Job drawing, mm, ordinate dimensions from the low corner. One solid piece. Coordinates: 2 decimals unless noted, no trailing zeros. Write each loop counter-clockwise with the first axis right and the second up, starting at its lowest first coordinate (ties: lowest second). Pieces come first, ordered by that corner, then holes. Notation, with made-up numbers: (-19, 63.5) - (13, 63.5) arc R30 cw to (13, 102.5) - close; hole circle Ø11 at (35.5, 5). An arc over 180 degrees is marked (long way). Use a Markdown table: item, result.
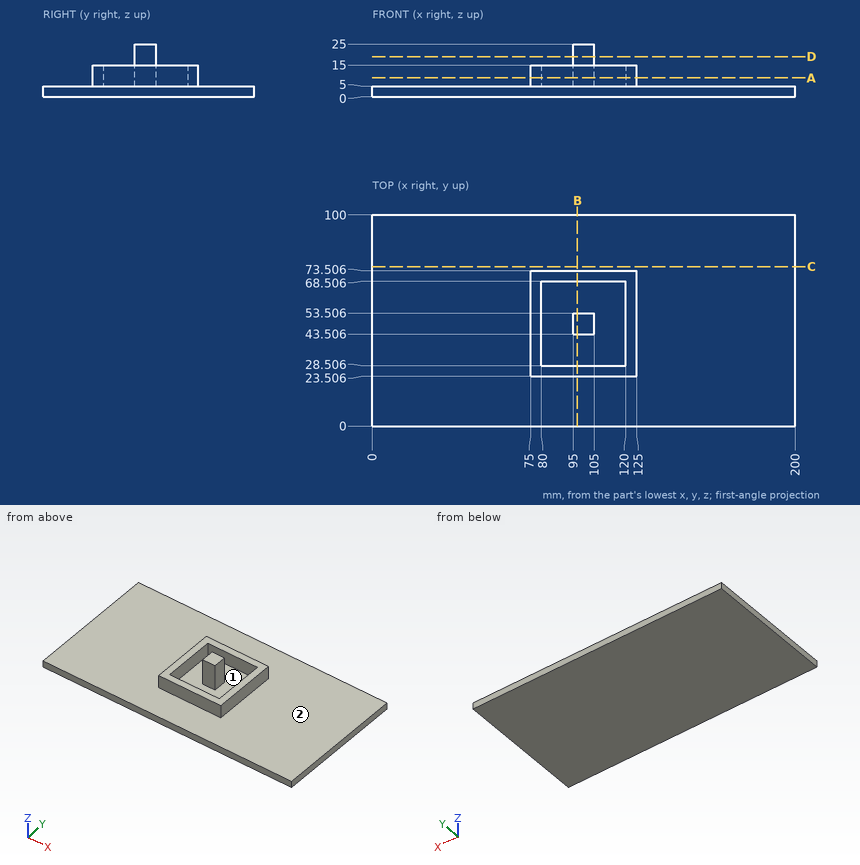
Item 1: Band-saw the part on D-D, the plane z = 19. Give the cut face in (x, y), then the cut area to 3 significant figures.
From the geometry:
| item | result |
|---|---|
| outline | (95, 43.51) - (105, 43.51) - (105, 53.51) - (95, 53.51) - close |
| area | 100 mm^2 |
Item 2: Drop flat-ended pins along their axis: P1, Ø8, axis at y = 71, z = 8, coming from the -X side; P2, Ø3, axis at x = 103.5, y = 61, coming from the +Z side; P3, Ø3, axis at y = 42.5, z = 9, coming from the +X side; P4, Ø8, axis at x = 103, z = 10, coming from the -Y side. Give the stop position or say it passes through.
From the geometry:
| item | result |
|---|---|
| P1 | x = 0 |
| P2 | z = 5 |
| P3 | x = 125 |
| P4 | y = 23.51 |
Item 3: Band-saw the part on C-C, the plane y = 75.5. Give the cut face in (x, z).
From the geometry:
| item | result |
|---|---|
| outline | (0, 0) - (200, 0) - (200, 5) - (0, 5) - close |
Item 4: Drill centre lines: probe 1 along X at (y, z) = (35.5, 5.5); probe 2 along Z at (x, y) = (115.5, 67.5); probe 3 along Y at (x, z) = (84.5, 13.75). Where is each one in solid material? Low to high.
From the geometry:
| item | result |
|---|---|
| probe 1 | 75 to 80, 120 to 125 |
| probe 2 | 0 to 5 |
| probe 3 | 23.51 to 28.51, 68.51 to 73.51 |
Item 5: Two-plate mould, pull along Y, no slides. Class the marked faces 1 and 2: pulls with the +Y half, pulls with the -Y half, needs draft (parallel to the pull), parting line crosses it, or undercut.
From the geometry:
| item | result |
|---|---|
| face 1 | undercut |
| face 2 | needs draft |
Item 6: Band-saw the part on A-A, the plane z = 9. Give the cut face in (x, y).
From the geometry:
| item | result |
|---|---|
| outline | (75, 23.51) - (125, 23.51) - (125, 73.51) - (75, 73.51) - close; (95, 43.51) - (105, 43.51) - (105, 53.51) - (95, 53.51) - close; hole (80, 28.51) - (120, 28.51) - (120, 68.51) - (80, 68.51) - close |
Item 7: Band-saw the part on B-B, the plane x = 97. Give the cut face in (y, z).
From the geometry:
| item | result |
|---|---|
| outline | (0, 0) - (100, 0) - (100, 5) - (73.51, 5) - (73.51, 15) - (68.51, 15) - (68.51, 5) - (53.51, 5) - (53.51, 25) - (43.51, 25) - (43.51, 5) - (28.51, 5) - (28.51, 15) - (23.51, 15) - (23.51, 5) - (0, 5) - close |
